from build123d import *

# Parameters (mm, degrees)
F2_W          = 55
F2_H          = 2.5
F4_DEPTH      = 40
F6_DEPTH      = 2.501
F6_DEPTH_BACK = 75
F8_DEPTH      = 2.501
F9_R          = 2.5


with BuildPart() as f4:
    # F2 (on Top) → F4 (new body)
    with BuildSketch(Plane.XY):
        with Locations((30, 40)):
            Rectangle(F2_W, F2_H)
        Polygon((0, 80), (0, 0), (60, 0), (60, 10), (57.5, 10), (57.5, 2.5), (2.5, 2.5), (2.5, 38.75), (2.5, 41.25), (2.5, 77.5), (57.5, 77.5), (57.5, 70), (60, 70), (60, 80), align=None)
    extrude(amount=F4_DEPTH)

    # F5 (on face) → F6 (cut, two sides)
    with BuildSketch(Plane.XZ.offset(-77.5)) as f6_sk:
        with BuildLine():
            ThreePointArc((18, 12), (23.6568542495, 14.3431457505), (26, 20))
            ThreePointArc((26, 20), (23.6568542495, 25.6568542495), (18, 28))
            ThreePointArc((18, 28), (10, 20), (18, 12))
        make_face()
        with BuildLine():
            ThreePointArc((18, 28), (23.6568542495, 25.6568542495), (26, 20))
            ThreePointArc((26, 20), (23.6568542495, 14.3431457505), (18, 12))
            Line((18, 12), (42, 12))
            ThreePointArc((42, 12), (34, 20), (42, 28))
            Line((42, 28), (18, 28))
        make_face()
        with BuildLine():
            ThreePointArc((50, 20), (47.6568542495, 25.6568542495), (42, 28))
            ThreePointArc((42, 28), (34, 20), (42, 12))
            ThreePointArc((42, 12), (47.6568542495, 14.3431457505), (50, 20))
        make_face()
    extrude(amount=-F6_DEPTH, mode=Mode.SUBTRACT)
    extrude(f6_sk.sketch, amount=F6_DEPTH_BACK, mode=Mode.SUBTRACT)

    # F7 (on face) → F8 (cut, through all)
    with BuildSketch(Plane(origin=(0, 2.5, 0), x_dir=(-1, 0, 0), z_dir=(0, 1, 0))):
        with BuildLine():
            ThreePointArc((-15.25, 30), (-14, 28.75), (-12.75, 30))
            ThreePointArc((-12.75, 30), (-14, 31.25), (-15.25, 30))
        make_face()
        with BuildLine():
            ThreePointArc((-15.25, 10), (-14, 11.25), (-12.75, 10))
            Line((-12.75, 10), (-12.75, 30))
            ThreePointArc((-12.75, 30), (-14, 28.75), (-15.25, 30))
            Line((-15.25, 30), (-15.25, 10))
        make_face()
        with BuildLine():
            ThreePointArc((-15.25, 10), (-14, 8.75), (-12.75, 10))
            ThreePointArc((-12.75, 10), (-14, 11.25), (-15.25, 10))
        make_face()
        with BuildLine():
            ThreePointArc((-19.25, 10), (-18, 8.75), (-16.75, 10))
            ThreePointArc((-16.75, 10), (-18, 11.25), (-19.25, 10))
        make_face()
        with BuildLine():
            ThreePointArc((-19.25, 10), (-18, 11.25), (-16.75, 10))
            Line((-16.75, 10), (-16.75, 30))
            ThreePointArc((-16.75, 30), (-18, 28.75), (-19.25, 30))
            Line((-19.25, 30), (-19.25, 10))
        make_face()
        with BuildLine():
            ThreePointArc((-19.25, 30), (-18, 28.75), (-16.75, 30))
            ThreePointArc((-16.75, 30), (-18, 31.25), (-19.25, 30))
        make_face()
        with BuildLine():
            ThreePointArc((-23.25, 30), (-22, 28.75), (-20.75, 30))
            ThreePointArc((-20.75, 30), (-22, 31.25), (-23.25, 30))
        make_face()
        with BuildLine():
            ThreePointArc((-23.25, 10), (-22, 11.25), (-20.75, 10))
            Line((-20.75, 10), (-20.75, 30))
            ThreePointArc((-20.75, 30), (-22, 28.75), (-23.25, 30))
            Line((-23.25, 30), (-23.25, 10))
        make_face()
        with BuildLine():
            ThreePointArc((-23.25, 10), (-22, 8.75), (-20.75, 10))
            ThreePointArc((-20.75, 10), (-22, 11.25), (-23.25, 10))
        make_face()
        with BuildLine():
            ThreePointArc((-27.25, 10), (-26, 8.75), (-24.75, 10))
            ThreePointArc((-24.75, 10), (-26, 11.25), (-27.25, 10))
        make_face()
        with BuildLine():
            ThreePointArc((-27.25, 30), (-26, 28.75), (-24.75, 30))
            ThreePointArc((-24.75, 30), (-26, 31.25), (-27.25, 30))
        make_face()
        with BuildLine():
            ThreePointArc((-31.25, 30), (-30, 28.75), (-28.75, 30))
            ThreePointArc((-28.75, 30), (-30, 31.25), (-31.25, 30))
        make_face()
        with BuildLine():
            Line((-28.75, 10), (-28.75, 30))
            ThreePointArc((-28.75, 30), (-30, 28.75), (-31.25, 30))
            Line((-31.25, 30), (-31.25, 10))
            ThreePointArc((-31.25, 10), (-30, 11.25), (-28.75, 10))
        make_face()
        with BuildLine():
            ThreePointArc((-31.25, 10), (-30, 8.75), (-28.75, 10))
            ThreePointArc((-28.75, 10), (-30, 11.25), (-31.25, 10))
        make_face()
        with BuildLine():
            ThreePointArc((-27.25, 10), (-26, 11.25), (-24.75, 10))
            Line((-24.75, 10), (-24.75, 30))
            ThreePointArc((-24.75, 30), (-26, 28.75), (-27.25, 30))
            Line((-27.25, 30), (-27.25, 10))
        make_face()
        with BuildLine():
            ThreePointArc((-32.75, 10), (-34, 11.25), (-35.25, 10))
            ThreePointArc((-35.25, 10), (-34, 8.75), (-32.75, 10))
        make_face()
        with BuildLine():
            ThreePointArc((-32.75, 30), (-34, 28.75), (-35.25, 30))
            Line((-35.25, 30), (-35.25, 10))
            ThreePointArc((-35.25, 10), (-34, 11.25), (-32.75, 10))
            Line((-32.75, 10), (-32.75, 30))
        make_face()
        with BuildLine():
            ThreePointArc((-32.75, 30), (-34, 31.25), (-35.25, 30))
            ThreePointArc((-35.25, 30), (-34, 28.75), (-32.75, 30))
        make_face()
        with BuildLine():
            ThreePointArc((-36.75, 30), (-38, 31.25), (-39.25, 30))
            ThreePointArc((-39.25, 30), (-38, 28.75), (-36.75, 30))
        make_face()
        with BuildLine():
            ThreePointArc((-36.75, 30), (-38, 28.75), (-39.25, 30))
            Line((-39.25, 30), (-39.25, 10))
            ThreePointArc((-39.25, 10), (-38, 11.25), (-36.75, 10))
            Line((-36.75, 10), (-36.75, 30))
        make_face()
        with BuildLine():
            ThreePointArc((-36.75, 10), (-38, 11.25), (-39.25, 10))
            ThreePointArc((-39.25, 10), (-38, 8.75), (-36.75, 10))
        make_face()
        with BuildLine():
            ThreePointArc((-40.75, 10), (-42, 11.25), (-43.25, 10))
            ThreePointArc((-43.25, 10), (-42, 8.75), (-40.75, 10))
        make_face()
        with BuildLine():
            ThreePointArc((-40.75, 30), (-42, 28.75), (-43.25, 30))
            Line((-43.25, 30), (-43.25, 10))
            ThreePointArc((-43.25, 10), (-42, 11.25), (-40.75, 10))
            Line((-40.75, 10), (-40.75, 30))
        make_face()
        with BuildLine():
            ThreePointArc((-40.75, 30), (-42, 31.25), (-43.25, 30))
            ThreePointArc((-43.25, 30), (-42, 28.75), (-40.75, 30))
        make_face()
        with BuildLine():
            ThreePointArc((-44.75, 30), (-46, 31.25), (-47.25, 30))
            ThreePointArc((-47.25, 30), (-46, 28.75), (-44.75, 30))
        make_face()
        with BuildLine():
            ThreePointArc((-44.75, 30), (-46, 28.75), (-47.25, 30))
            Line((-47.25, 30), (-47.25, 10))
            ThreePointArc((-47.25, 10), (-46, 11.25), (-44.75, 10))
            Line((-44.75, 10), (-44.75, 30))
        make_face()
        with BuildLine():
            ThreePointArc((-44.75, 10), (-46, 11.25), (-47.25, 10))
            ThreePointArc((-47.25, 10), (-46, 8.75), (-44.75, 10))
        make_face()
    extrude(amount=-F8_DEPTH, mode=Mode.SUBTRACT)

    # F9
    f9_edges = [f4.edges().sort_by_distance(p)[0] for p in [
        (2.5, 41.25, 20),
        (2.5, 38.75, 20),
        (2.5, 77.5, 20),
        (60, 80, 20),
        (57.5, 77.5, 20),
        (0, 80, 20),
        (2.5, 2.5, 20),
        (57.5, 2.5, 20),
        (0, 0, 20),
        (60, 0, 20),
    ]]
    fillet(f9_edges, radius=F9_R)


solid = f4.part
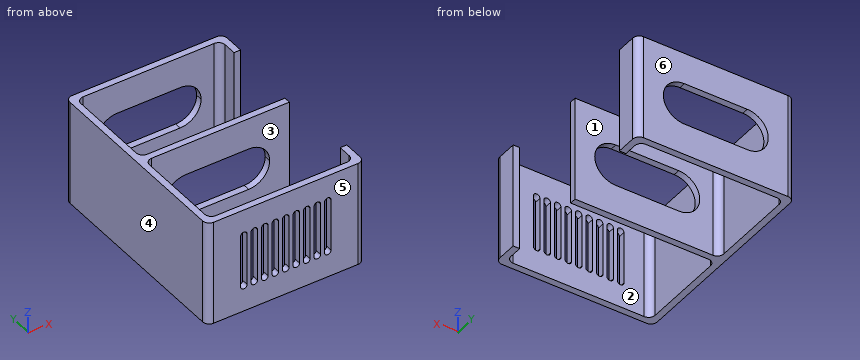
Work out the finished part from the listing and answer in its coordinate system (mm). Face numbers are marked on the shaded views. A direction names the side the tool comes from. Coordinates: 2 decimals unless noted, no trailing zeros. Write each loop counter-clockwise with the first axis right and the second up, starting at its lowest first coordinate (ties: lowest second). Pieces come first, ordered by that corner, then holes. Notation, with made-up numbers: M -10,-19.5 L 30,-19.5 A13 cw 30,-4.5 Z; hole C 81.5,19 d4. An arc over 180 degrees is marked long. Answer as CSV lines item,"result". Start each with the question number.
Item 1: Section D-D on z = 17 is taken. Give the number of separate pieces and of enclosed holes in the cut face, and give its area (3 significant figures).
Item 2: Consider L1, parallel to Y at x = 39.5, z = 31.5; L2, parallel to Y at x = 41.5, z = 9.5; L3, parallel to X at y = 72, z = 6.5. Determine where each line is inside the solid, lowest interval first.
Item 3: Determine the mould class of the marked faces 3, 4, 5 and 6 for opening direction Y: released by +Y, released by -Y, zero draft, split by the parting line, or undercut.
Item 4: Section A-A on x = 34 is taken. Write down the section's boundary in (y, z), and give its area (3 significant figures).
Item 5: Section C-C on y = 50.5 is taken. Write down the section's boundary in (x, z).
Item 6: A tool of negligible diameter and unlimited length cuts with its end or side. For the marked faces 1 and 2, from which of +Z, -Z, +X, -X, +Y, -Y can it reach the whole face along a straight path? Write none if from no direction.
Item 7: Section B-B on z = 3 is taken. Write down the section's boundary in (x, y), and give its area (3 significant figures).
Item 8: Flat-ended cylindrical pins translate along their axes: P1, Ø5, axis at y = 32, z = 12, coming from the +X side; P2, Ø10, axis at x = 13.5, y = 69.5, coming from the +Z side (1 decimal); P3, Ø2, axis at y = 1, z = 22, coming from the -X side; P4, Ø0.8, axis at y = 1, z = 22.5, coming from the +X side (3 decimals). Find the tip coordinate at first contact, or state that the pin passes through.
Checks:
1,separate pieces,"12"
1,enclosed holes,"0"
1,area,"415 mm²"
2,L1,"y = 0 to 2.5, 38.75 to 41.25, 77.5 to 80"
2,L2,"y = 38.75 to 41.25, 77.5 to 80"
2,L3,"x = 0 to 2.5, 57.5 to 60"
3,face 3,"undercut"
3,face 4,"zero draft"
3,face 5,"released by -Y"
3,face 6,"released by +Y"
4,outline,"M 0,0 L 2.5,0 L 2.5,8.75 L 0,8.75 Z; M 0,31.25 L 2.5,31.25 L 2.5,40 L 0,40 Z; M 38.75,0 L 41.25,0 L 41.25,12 L 38.75,12 Z; M 38.75,28 L 41.25,28 L 41.25,40 L 38.75,40 Z; M 77.5,0 L 80,0 L 80,12 L 77.5,12 Z; M 77.5,28 L 80,28 L 80,40 L 77.5,40 Z"
4,area,"164 mm²"
5,outline,"M 0,0 L 2.5,0 L 2.5,40 L 0,40 Z"
6,face 1,"+Z, -Z, +X"
6,face 2,"+Z, -Z"
7,outline,"M 0,2.5 A2.5 ccw 2.5,0 L 57.5,0 A2.5 ccw 60,2.5 L 60,10 L 57.5,10 L 57.5,5 A2.5 cw 55,2.5 L 5,2.5 A2.5 cw 2.5,5 L 2.5,36.25 A2.5 cw 5,38.75 L 57.5,38.75 L 57.5,41.25 L 5,41.25 A2.5 cw 2.5,43.75 L 2.5,75 A2.5 cw 5,77.5 L 55,77.5 A2.5 cw 57.5,75 L 57.5,70 L 60,70 L 60,77.5 A2.5 ccw 57.5,80 L 2.5,80 A2.5 ccw 0,77.5 Z"
7,area,"665 mm²"
8,P1,"stops at x = 2.5"
8,P2,"passes through"
8,P3,"stops at x = 0.05"
8,P4,"stops at x = 59.745"
